```python
from build123d import *

# Parameters (mm, degrees)
F0_W = 7.6932697557
F0_H = 49.7964322567
F2_T = -2.54
F3_R = 2.53999


# Not quite as in the source:
# - a fillet or chamfer is up to 0.001 mm smaller than in the source, because OpenCascade refuses the exact size


with BuildPart() as f1:
    # F0 (on Front) → F1 (revolve)
    with BuildSketch(Plane.XZ):
        with Locations((3.8466348778, 4.3362062424)):
            Rectangle(F0_W, F0_H)
    revolve(axis=Axis((0, 0, 4.3362062424), (0, 0, -1)))

    # F2
    f2_openings = [f1.faces().sort_by_distance(p)[0] for p in [
        (0, 0, 29.234422),
        (0, 0, -20.56201),
    ]]
    offset(amount=F2_T, openings=f2_openings)

    # F3 (radius 2.54 in the source; OpenCascade refuses exactly that, so slightly less here)
    f3_edges = [f1.edges().sort_by_distance(p)[0] for p in [
        (-7.69327, 0, -20.56201),
    ]]
    fillet(f3_edges, radius=F3_R)


solid = f1.part
```
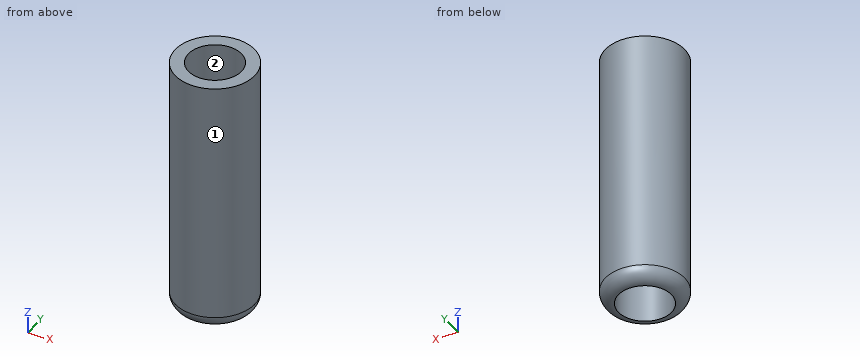
For this review, take the finished solid that the model builds, in its own axes (mm). Face numbers are marked on the shaded views. Give positions to 0.01 mm unless a question says otherwise; leave off trailing zeros. Order: outer loops, then holes, each group sorted by start corner. A loop starts at its lowest first (then second) coordinate and runs counter-clockwise, first axis right, second up.
1) Wall thickness on line 1 (X direction, y = 0, z = 12): over which ranges is the line inside the solid? List them lowest first.
2) Take a section at C-C (z = 22). Give the boundary of the cut face in (x, y).
3) Insertion check: pin 1 (1 mm diameter, centred on y = -5.5, z = 12, fed in from -X); pin 2 (8 mm diameter, centred on x = 4.5, z = -10, fed in from -Y); pin 3 (5 mm diameter, centred on x = 1, y = 0, fed in from -Z); pin 4 (5 mm diameter, centred on y = -5.5, z = 16.5, fed in from -X). Each pin has a flat end and moves straight along its axis. Give the tip position at first contact, or say it passes through.
4) The part is to be moulded in two halves that separate along X. For the marked faces 1 and 2, say which applies: released by +X, released by -X, zero draft, split by the parting line, or undercut.
Derived:
1. line 1: x = -7.69 to -5.15, 5.15 to 7.69
2. outline: circle Ø15.39 at (0, 0); hole circle Ø10.31 at (0, 0)
3. pin 1: stops at x = -5.85
3. pin 2: stops at y = -7.68
3. pin 3: passes through
3. pin 4: stops at x = -7.08
4. face 1: split by the parting line
4. face 2: undercut
